from build123d import *

# Parameters (mm, degrees)
BOSS_EXTRUDE1_DEPTH     = 203.2
SKETCH2_W               = 165.1
SKETCH2_H               = 165.1
CUT_EXTRUDE1_DEPTH      = 1
CUT_EXTRUDE1_DEPTH_BACK = 1874.504


with BuildPart() as part:
    # Sketch1 → Boss-Extrude1 (new body)
    with BuildSketch(Plane.XY):
        Polygon((0, 0), (203.2, 0), (203.2, 1873.504), (0, 1472.107144898), align=None)
    extrude(amount=BOSS_EXTRUDE1_DEPTH)

    # Sketch2 → Cut-Extrude1 (cut, two sides)
    with BuildSketch(Plane.XZ) as cut_extrude1_sk:
        with Locations((101.6, 101.6)):
            Rectangle(SKETCH2_W, SKETCH2_H)
    extrude(amount=CUT_EXTRUDE1_DEPTH, mode=Mode.SUBTRACT)
    extrude(cut_extrude1_sk.sketch, amount=-CUT_EXTRUDE1_DEPTH_BACK, mode=Mode.SUBTRACT)


solid = part.part
Could you check a few things on this model? Use its own coordinates, in mm. A direction names the side the tool comes from. Coordinates: 2 decimals unless noted, no trailing zeros. Write each loop counter-clockwise with the first axis right and the second up, starting at its lowest first coordinate (ties: lowest second). Pieces come first, ordered by that corner, then holes. Notation, with made-up numbers: (-21.5, 54.5) - (-13.5, 54.5) arc R33 cw to (-13.5, 87.5) - close; hole circle Ø3 at (-6.75, -1.75). An arc over 180 degrees is marked (long way). Put each result on its own line as item: value. Start each with the question number.
Q1. Which directions (+Z, -Z, +X, -X, +Y, -Y) give clear straight access to the entire face, cutting with the end or side of a thin tool? Please do faces 1 (the flat face through (203.2, 924, 100)), 2 (the flat face through (100, 905, 184.15)).
Q2. I want a section at C-C on y = 1169. Write out the boundary of the cut face in (x, z), plus the area to 3 significant figures.
Q3. Thinking about a two-plate mould opening in X: for faces 3 (the flat face through (100, 950, 203.2)), 4 (the flat face through (19.05, 744, 100)), 5 (the flat face through (103.022, 1675.615, 190.489)), which applies, pulls with the +X half, pulls with the -X half, needs draft (parallel to the pull), parting line crosses it, or undercut?
Q4. I want a section at B-B on x = 117.5. Write out the boundary of the cut face in (y, z).
Q5. Please list where these lines run through material, in increasing order: L1, parallel to Z at x = 95.5, y = 826; L2, parallel to X at y = 1762, z = 33.5.
Q6. I want a section at D-D on y = 1761. Write out the boundary of the cut face in (x, z).
Q7. I want a section at A-A on z = 128. Write out the boundary of the cut face in (x, y), plus the area to 3 significant figures.
Checks:
1. face 1: +Z, -Z, +X, +Y, -Y
1. face 2: +Y, -Y
2. outline: (0, 0) - (203.2, 0) - (203.2, 203.2) - (0, 203.2) - close; hole (19.05, 19.05) - (184.15, 19.05) - (184.15, 184.15) - (19.05, 184.15) - close
2. area: 14,000 mm²
3. face 3: needs draft
3. face 4: undercut
3. face 5: pulls with the -X half
4. outline: (0, 0) - (1704.21, 0) - (1704.21, 19.05) - (0, 19.05) - close; (0, 184.15) - (1704.21, 184.15) - (1704.21, 203.2) - (0, 203.2) - close
5. L1: 0 to 19.05, 184.15 to 203.2
5. L2: 184.15 to 203.2
6. outline: (146.25, 0) - (203.2, 0) - (203.2, 203.2) - (146.25, 203.2) - (146.25, 184.15) - (184.15, 184.15) - (184.15, 19.05) - (146.25, 19.05) - close
7. outline: (0, 0) - (19.05, 0) - (19.05, 1509.74) - (0, 1472.11) - close; (184.15, 0) - (203.2, 0) - (203.2, 1873.5) - (184.15, 1835.87) - close
7. area: 63,700 mm²
